from build123d import *

# Parameters (mm, degrees)
F0_R     = 14
F1_DEPTH = 10
F2_R     = 5
F2_R_2   = 1.5
F3_DEPTH = 2
F4_DEPTH = 10
F5_W     = 5
F5_H     = 1.524
F6_DEPTH = 2
F7_R     = 1.5
F8_DEPTH = 25.4
F9_R     = 1.5


# Not quite as in the source:
# - a pattern or mirror of a feature is missing from the dataset's text; its kind, count and spacing are read off the source's solid


with BuildPart() as f1:
    # F0 (on Top) → F1 (new body)
    with BuildSketch(Plane.XY):
        Circle(F0_R)
    extrude(amount=F1_DEPTH)

    # F2 (on face) → F3 (join)
    with BuildSketch(Plane.XY.offset(10)):
        Circle(F2_R)
        Circle(F2_R_2, mode=Mode.SUBTRACT)
    extrude(amount=F3_DEPTH)

    # F4 (add): a face of the model
    f4_faces = [f1.faces().sort_by_distance(p)[0] for p in [
        (0, 0, 10),
    ]]
    extrude(f4_faces, amount=F4_DEPTH)

    # F5 (on Front) → F6 (join, symmetric)
    with BuildSketch(Plane.XZ):
        Polygon((14, 0), (-14, 0), (-14, -1.524), (-12.476, -1.524), (12.476, -1.524), (14, -1.524), align=None)
        Polygon((-12.476, -1.524), (-14, -1.524), (-14, -1.651), (-14, -3.175), (-12.476, -3.175), align=None)
        with Locations((-16.5, -2.413)):
            Rectangle(F5_W, F5_H)
        Polygon((14, -1.651), (14, -1.524), (12.476, -1.524), (12.476, -3.175), (14, -3.175), align=None)
        with Locations((16.5, -2.413)):
            Rectangle(F5_W, F5_H)
    f6 = extrude(amount=F6_DEPTH, both=True)

    # F6_copies: F6 across plane
    add(f6.mirror(Plane(origin=(0, 0, 0), x_dir=(-0.7071067812, -0.7071067812, 0), z_dir=(-0.7071067812, 0.7071067812, 0))))

    # F7 (on face) → F8 (cut)
    with BuildSketch(Plane.XY.offset(-1.651)):
        with Locations((-16.5, 0)):
            Circle(F7_R)
        with BuildLine():
            ThreePointArc((18, 0), (16.5, 1.5), (15, 0))
            ThreePointArc((15, 0), (16.5, -1.5), (18, 0))
        make_face()
    f8 = extrude(amount=-F8_DEPTH, mode=Mode.SUBTRACT)

    # F8_copies: F8 across plane
    add(f8.mirror(Plane(origin=(0, 0, 0), x_dir=(0.7071067812, 0.7071067812, 0), z_dir=(0.7071067812, -0.7071067812, 0))), mode=Mode.SUBTRACT)

    # F9
    f9_edges = [f1.edges().sort_by_distance(p)[0] for p in [
        (-19, -2, -2.413),
        (-19, 2, -2.413),
        (19, -2, -2.413),
        (19, 2, -2.413),
        (2, 19, -2.413),
        (-2, 19, -2.413),
        (-2, -19, -2.413),
        (2, -19, -2.413),
    ]]
    fillet(f9_edges, radius=F9_R)


solid = f1.part
Source: CAD feature listing. Evaluate the final solid. Frame: model axes, mm. A direction names the side the tool comes from. Round coordinates to 2 decimals unless told otherwise and drop trailing zeros. Loops run counter-clockwise (first coordinate to the right, second up) from the corner with the lowest first, then second, coordinate; pieces in that order, holes last. Notation, with made-up numbers: M -4,33.5 L 28,33.5 A15 cw 28,62.5 Z; hole C 7.25,15 d9. An arc over 180 degrees is marked long. Return JSON: item names as keys, results as strings. Group by question number.
1. Material intervals for line 1 along X through (y, z) = (16.5, -2.4); line 2 along Y through (x, z) = (10, -0.5), sorted ascending. Write a range as from..to.
2. Section query D-D on y = 2.5. Output: boundary loops of the cut face in (x, z).
3. Section query C-C on x = -1. State how many separate pieces and enclosed holes the cut face has, and give its area (3 significant figures).
4. Pin query (flat end, axial travel): pin 1 (3.5 mm diameter, centred on y = -11, z = -2, fed in from +X); pin 2 (2.5 mm diameter, centred on x = -16.5, y = 0, fed in from +Z); pin 3 (1.5 mm diameter, centred on x = 4, y = 8, fed in from -Z); pin 4 (5 mm diameter, centred on y = -10.5, z = 1, fed in from +X). Return the tip coordinate at first contact, or that it passes through.
5. Mould query, pull axis Y, two halves, no side actions, for faces 1 (the face through (-18.55, -1.57, -2.4)), 2 (the face through (0, 0, 20)), 3 (the face through (18, 0, -2)). Classes: released by +Y, released by -Y, zero draft, split by the parting line, or undercut.
6. Reachability of faces 4 (the face through (2, -10, -1)), 5 (the face through (-14, 0, -1)), 6 (the face through (-2, -10, -1)) from +Z, -Z, +X, -X, +Y, -Y: full face, straight path, thin tool, end or side. Return the list, or none.
7. Section query A-A on y = 16.5. Output: boundary loops of the cut face in (x, z) (3 decimals), and give its area (3 significant figures).
Checks:
{
 "1": {"line 1": "x = -2..-1.5, 1.5..2", "line 2": "y = -2..2"},
 "2": {"outline": "M -13.77,0 L -2,0 L -2,-1.52 L 2,-1.52 L 2,0 L 13.77,0 L 13.77,10 L 4.33,10 L 4.33,12 L -4.33,12 L -4.33,10 L -13.77,10 Z"},
 "3": {"separate pieces": "3", "enclosed holes": "0", "area": "373 mm²"},
 "4": {"pin 1": "stops at x = 2", "pin 2": "passes through", "pin 3": "stops at z = 0", "pin 4": "stops at x = 11.49"},
 "5": {"face 1": "released by -Y", "face 2": "zero draft", "face 3": "undercut"},
 "6": {"face 4": "-Z, +X, -Y", "face 5": "+Z, -X, +Y, -Y", "face 6": "-Z, -X, -Y"},
 "7": {"outline": "M -2,-3.175 L -1.5,-3.175 L -1.5,-1.651 L -2,-1.651 Z; M 1.5,-3.175 L 2,-3.175 L 2,-1.651 L 1.5,-1.651 Z", "area": "1.52 mm²"}
}
